Geometry check sheet. Reference: drawing and pictorial views, mm from the part's lowest x, y, z. Round coordinates to 2 decimals unless told otherwise and drop trailing zeros. Order: outer loops, then holes, each group sorted by start corner. A loop starts at its lowest first (then second) coordinate and runs counter-clockwise, first axis right, second up.
(1) Sectioned sample at C-C (z = 691). Record the boundary of the cut face in (x, y).
(2) Sectioned sample at B-B (z = 295). Record the boundary of the cut face in (x, y) (1 decimal).
(3) Go/stop test with flat-tipped pins: pin 1 (5 mm diameter, centred on y = 263, z = 511, fed in from -X); pin 2 (12 mm diameter, centred on x = 335, z = 268, fed in from +Y) (1 decimal); pin 3 (1.5 mm diameter, centred on x = 359, z = 519, fed in from +Y). Record where each tip stops, or that it passes through.
(4) Release check for a two-part mould opening along X. For the marked faces 1, 2 and 3 record: +X half, -X half, draft (parallel to the pull), parting line (faces both ways), or undercut.
(5) Sectioned sample at A-A (x = 200). Record the boundary of the cut face in (y, z), plus the area to 3 significant figures.
(6) Material ranges on line 1 along Z through (x, y) = (86.5, 245); line 2 along X through (y, z) = (102, 126); line 3 along Y through (x, z) = (77.5, 594), recorded low to high.
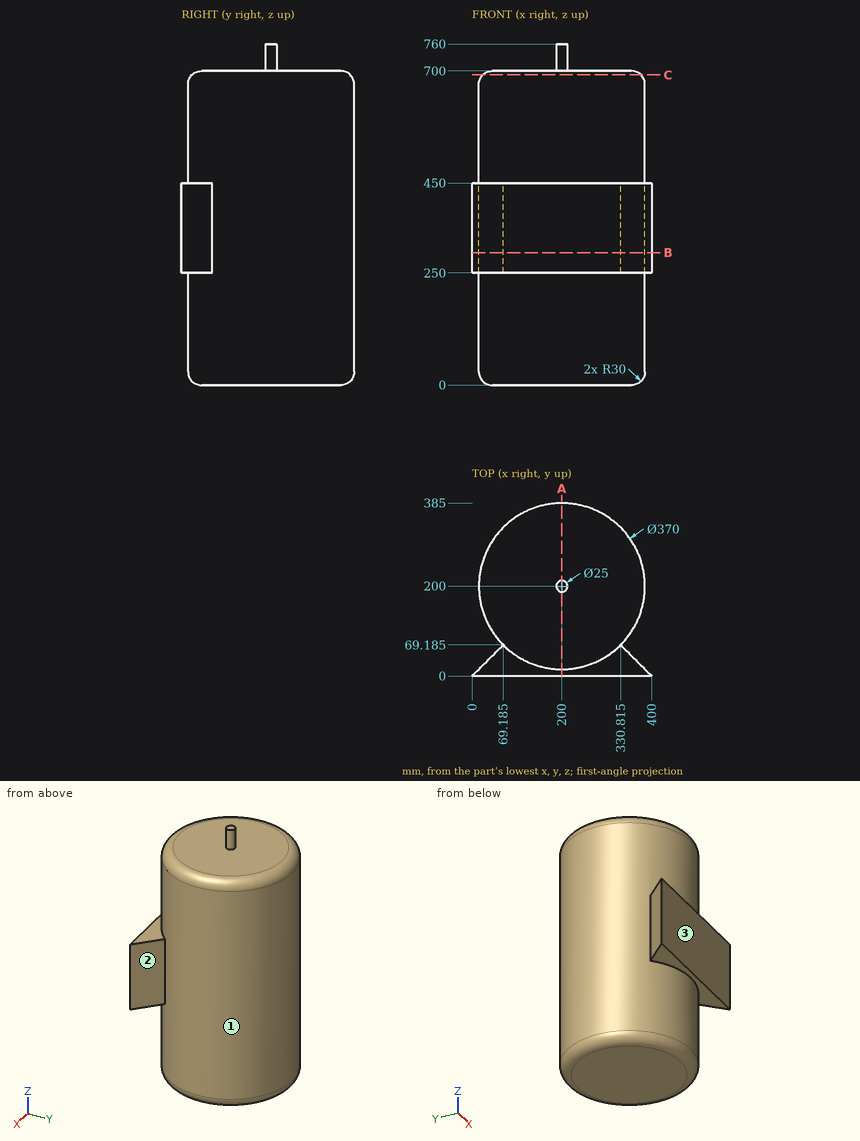
Answer below:
1. outline: circle Ø352.85 at (200, 200)
2. outline: (0, 0) - (400, 0) - (330.8, 69.2) arc R185 ccw (long way) to (69.2, 69.2) - close
3. pin 1: stops at x = 25.17
3. pin 2: stops at y = 332.6
3. pin 3: stops at y = 295.82
4. face 1: parting line
4. face 2: +X half
4. face 3: draft
5. outline: (0, 250) - (15, 250) - (15, 30) arc R30 ccw to (45, 0) - (355, 0) arc R30 ccw to (385, 30) - (385, 670) arc R30 ccw to (355, 700) - (212.5, 700) - (212.5, 760) - (187.5, 760) - (187.5, 700) - (45, 700) arc R30 ccw to (15, 670) - (15, 450) - (0, 450) - close
5. area: 263,000 mm2
6. line 1: z = 0 to 700
6. line 2: x = 43.09 to 356.91
6. line 3: y = 61.37 to 338.63
